from build123d import *

# Parameters (mm, degrees)
SKETCH_1_W                       = 120
SKETCH_1_H                       = 88
SKETCH_1_R                       = 32.5
SM_BASE_FLANGE_1_DEPTH           = 6
SM_EDGE_FLANGE_5_STRIP_W         = 36
SM_EDGE_FLANGE_5_STRIP_H         = 6
SM_EDGE_FLANGE_5_STRIP_CUT_DEPTH = 88
SM_EDGE_FLANGE_5_DEPTH           = 88
SM_EDGE_FLANGE_7_DEPTH           = 108
OTHER_START                      = -12
OTHER_1_OUTLINE_W                = 12
OTHER_1_OUTLINE_H                = 63
OTHER_1_DEPTH                    = 6
OTHER_START_2                    = -5
OTHER_1_2_OUTLINE_W              = 6
OTHER_1_2_OUTLINE_H              = 63
OTHER_1_2_DEPTH                  = 5
CHAMFER_1_SIZE                   = 25
MOVE_START                       = -12
MOVE_BODY_1_DEPTH                = 100
MOVE_START_2                     = -5
MOVE_BODY_1_2_OUTLINE_W          = 108
MOVE_BODY_1_2_OUTLINE_H          = 12
MOVE_BODY_1_2_OUTLINE_W_2        = 6
MOVE_BODY_1_2_OUTLINE_H_2        = 63
MOVE_BODY_1_2_DEPTH              = 93
MOVE_BODY_1_3_DEPTH              = 6
MOVE_BODY_1_4_DEPTH              = 88
MOVE_START_3                     = -6
MOVE_BODY_1_5_OUTLINE_W          = 108
MOVE_BODY_1_5_OUTLINE_H          = 12
MOVE_BODY_1_5_DEPTH              = 1
MOVE_BODY_1_6_OUTLINE_R          = 32.5
MOVE_BODY_1_6_DEPTH              = 12
MOVE_BODY_1_7_DEPTH              = 108


with BuildPart() as part:
    # Базовая кромка1: sheet metal written as solids
    # Sketch 1 → Базовая кромка1 (new body)
    with BuildSketch(Plane.XY):
        with Locations((60, 44)):
            Rectangle(SKETCH_1_W, SKETCH_1_H)
        with Locations((60, 38)):
            Circle(SKETCH_1_R, mode=Mode.SUBTRACT)
    extrude(amount=-SM_BASE_FLANGE_1_DEPTH)

    # Ребро-кромка5: sheet metal written as solids
    # Ребро-кромка5 strip (on a plane across the edge) → Ребро-кромка5 strip cut (cut)
    with BuildSketch(Plane(origin=(120, 0, 0), x_dir=(-1, 0, 0), z_dir=(0, 1, 0))):
        with Locations((-6, -3)):
            Rectangle(SM_EDGE_FLANGE_5_STRIP_W, SM_EDGE_FLANGE_5_STRIP_H)
    extrude(amount=SM_EDGE_FLANGE_5_STRIP_CUT_DEPTH, mode=Mode.SUBTRACT)

    # Ребро-кромка5 section (on a plane across the edge) → Ребро-кромка5 (add)
    with BuildSketch(Plane(origin=(120, 0, 0), x_dir=(-1, 0, 0), z_dir=(0, 1, 0))):
        with BuildLine():
            Line((0, 6), (0, 69))
            Line((0, 69), (6, 69))
            Line((6, 69), (6, 6))
            ThreePointArc((6, 6), (7.757359313, 1.757359313), (12, 0))
            Line((12, 0), (12, -6))
            ThreePointArc((12, -6), (3.514718626, -2.485281374), (0, 6))
        make_face()
    extrude(amount=SM_EDGE_FLANGE_5_DEPTH)

    # Ребро-кромка7: sheet metal written as solids
    # Ребро-кромка7 section (on a plane across the edge) → Ребро-кромка7 (add)
    with BuildSketch(Plane(origin=(0, -6, 0), x_dir=(0, 1, 0), z_dir=(1, 0, 0))):
        with BuildLine():
            Line((-6, 6), (-6, 69))
            Line((-6, 69), (0, 69))
            Line((0, 69), (0, 6))
            ThreePointArc((0, 6), (1.757359313, 1.757359313), (6, 0))
            Line((6, 0), (6, -6))
            ThreePointArc((6, -6), (-2.485281374, -2.485281374), (-6, 6))
        make_face()
    extrude(amount=SM_EDGE_FLANGE_7_DEPTH)

    # Other 1: read off the stored shape, not the designer's step
    # Other 1 outline → Other 1 (add)
    with BuildSketch(Plane(origin=(0, 0, 0), x_dir=(1, 0, 0), z_dir=(0, 1, 0)).offset(OTHER_START)):
        with Locations((114, -37.5)):
            Rectangle(OTHER_1_OUTLINE_W, OTHER_1_OUTLINE_H)
    extrude(amount=OTHER_1_DEPTH)

    # Other 1 2 outline → Other 1 2 (add)
    with BuildSketch(Plane(origin=(0, 0, 0), x_dir=(1, 0, 0), z_dir=(0, 1, 0)).offset(OTHER_START_2)):
        with Locations((117, -37.5)):
            Rectangle(OTHER_1_2_OUTLINE_W, OTHER_1_2_OUTLINE_H)
    extrude(amount=OTHER_1_2_DEPTH)

    # Фаска1
    chamfer_1_edges = [part.edges().sort_by_distance(p)[0] for p in [
        (0, -9, 69),
        (0, 88, -3),
    ]]
    chamfer(chamfer_1_edges, length=CHAMFER_1_SIZE)

    # Move Body 1: read off the stored shape, not the designer's step
    # Move Body 1 outline → Move Body 1 (cut)
    with BuildSketch(Plane(origin=(0, 0, 0), x_dir=(1, 0, 0), z_dir=(0, 1, 0)).offset(MOVE_START)):
        with BuildLine():
            Line((0, -6), (0, -44))
            Line((0, -44), (25, -69))
            Line((25, -69), (120, -69))
            Line((120, -69), (120, -6))
            ThreePointArc((120, -6), (119.591109915, -2.894171459), (118.392304845, 0))
            ThreePointArc((118.392304845, 0), (116.40755123, -2.562305899), (113.809475019, -4.5))
            ThreePointArc((113.809475019, -4.5), (113.952178178, -5.243974245), (114, -6))
            Line((114, -6), (0, -6))
        make_face()
        with BuildLine():
            Line((108, 6), (108, 0))
            ThreePointArc((108, 0), (111.674234614, 1.25658351), (113.809475019, 4.5))
            ThreePointArc((113.809475019, 4.5), (111, 5.618950038), (108, 6))
        make_face()
    extrude(amount=MOVE_BODY_1_DEPTH, mode=Mode.SUBTRACT)

    # Move Body 1 2 outline → Move Body 1 2 (add)
    with BuildSketch(Plane(origin=(0, 0, 0), x_dir=(1, 0, 0), z_dir=(0, 1, 0)).offset(MOVE_START_2)):
        with Locations((54, 0)):
            Rectangle(MOVE_BODY_1_2_OUTLINE_W, MOVE_BODY_1_2_OUTLINE_H)
        with Locations((117, 37.5)):
            Rectangle(MOVE_BODY_1_2_OUTLINE_W_2, MOVE_BODY_1_2_OUTLINE_H_2)
    extrude(amount=MOVE_BODY_1_2_DEPTH)

    # Move Body 1 3 outline → Move Body 1 3 (add)
    with BuildSketch(Plane(origin=(0, 0, 0), x_dir=(1, 0, 0), z_dir=(0, 1, 0)).offset(MOVE_START)):
        Polygon((0, -6), (108, -6), (108, 6), (120, 6), (120, 69), (25, 69), (0, 44), align=None)
    extrude(amount=MOVE_BODY_1_3_DEPTH)

    # Move Body 1 4 outline → Move Body 1 4 (add)
    with BuildSketch(Plane(origin=(0, 0, 0), x_dir=(1, 0, 0), z_dir=(0, 1, 0))):
        with BuildLine():
            Line((108, 0), (108, -6))
            ThreePointArc((108, -6), (111, -5.618950038), (113.809475019, -4.5))
            ThreePointArc((113.809475019, -4.5), (111.674234614, -1.25658351), (108, 0))
        make_face()
        with BuildLine():
            ThreePointArc((113.809475019, 4.5), (116.40755123, 2.562305899), (118.392304845, 0))
            ThreePointArc((118.392304845, 0), (119.591109915, 2.894171459), (120, 6))
            Line((120, 6), (114, 6))
            ThreePointArc((114, 6), (113.952178178, 5.243974245), (113.809475019, 4.5))
        make_face()
    extrude(amount=MOVE_BODY_1_4_DEPTH)

    # Move Body 1 5 outline → Move Body 1 5 (add)
    with BuildSketch(Plane(origin=(0, 0, 0), x_dir=(1, 0, 0), z_dir=(0, 1, 0)).offset(MOVE_START_3)):
        with Locations((54, 0)):
            Rectangle(MOVE_BODY_1_5_OUTLINE_W, MOVE_BODY_1_5_OUTLINE_H)
    extrude(amount=MOVE_BODY_1_5_DEPTH)

    # Move Body 1 6 outline → Move Body 1 6 (cut)
    with BuildSketch(Plane.XY.offset(MOVE_START_3)):
        with Locations((60, 38)):
            Circle(MOVE_BODY_1_6_OUTLINE_R)
        Polygon((0, 88), (0, 63), (25, 88), align=None)
    extrude(amount=MOVE_BODY_1_6_DEPTH, mode=Mode.SUBTRACT)

    # Move Body 1 7 outline → Move Body 1 7 (cut)
    with BuildSketch(Plane.YZ):
        with BuildLine():
            Line((88, -6), (88, 0))
            Line((88, 0), (0, 0))
            ThreePointArc((0, 0), (-4.242640687, -1.757359313), (-6, -6))
            Line((-6, -6), (88, -6))
        make_face()
        with BuildLine():
            ThreePointArc((-12, -6), (-8.485281374, 2.485281374), (0, 6))
            Line((0, 6), (-12, 6))
            Line((-12, 6), (-12, -6))
        make_face()
    extrude(amount=MOVE_BODY_1_7_DEPTH, mode=Mode.SUBTRACT)


solid = part.part
Geometry: final body of the model. Coordinates: model frame, mm. A direction names the side the tool comes from. Give positions to 0.01 mm unless a question says otherwise; leave off trailing zeros. Loops run counter-clockwise (first coordinate to the right, second up) from the corner with the lowest first, then second, coordinate; pieces in that order, holes last. Notation, with made-up numbers: M 18.5,62.5 L 47.5,62.5 A32 cw 47.5,89.5 Z; hole C -34.75,79 d4. An arc over 180 degrees is marked long. Put each result on its own line as item: value.
1) Cut plane A-A, the plane x = 60. Return the cut outline in (y, z).
Computed values:
outline: M -12,-69 L -6,-69 L -6,-6 A6 cw 0,0 L 5.5,0 L 5.5,6 L 0,6 A12 ccw -12,-6 Z; M 70.5,0 L 88,0 L 88,6 L 70.5,6 Z
2) First-contact query: P1, Ø4, axis at x = 118.5, y = -1.5, coming from the +Z side; P2, Ø6.5, axis at x = 115, y = -7.5, coming from the +Z side; P3, Ø9.5, axis at x = 111, z = 0.5, coming from the -Y side. Flat tips, straight axial feed; report the tip coordinate or a pass-through.
Computed values:
P1: stops at z = 1.73
P2: stops at z = -6
P3: stops at y = -11.66
3) Reachability of faces 1 (the flat face through (29, 54, 0)), 2 (the flat face through (59, -12, -38)), 3 (the flat face through (108, -6, 0)) from +Z, -Z, +X, -X, +Y, -Y: full face, straight path, thin tool, end or side. Return the list, or none.
Computed values:
face 1: -Z, -X, +Y
face 2: +Z, -Z, +X, -X, -Y
face 3: +Z, +X, -Y
4) Cut plane D-D, the plane y = 3. Return the cut outline in (x, z), plus the area to 3 significant figures.
Computed values:
outline: M 0,0 L 108,0 A6 cw 114,-6 L 114,-69 L 120,-69 L 120,-6 A12 ccw 108,6 L 0,6 Z
area: 1,110 mm^2
5) Mould query, pull axis Y, two halves, no side actions, for faces 4 (the flat face through (29, 53, 6)), 5 (the flat face through (93, 88, 2)), 6 (the flat face through (117, -5, -38)), 7 (the cylindrical face through (27.53, 39.43, 2.96)). Classes: released by +Y, released by -Y, zero draft, split by the parting line, or undercut.
Computed values:
face 4: zero draft
face 5: released by +Y
face 6: undercut
face 7: undercut
6) Cut plane C-C, the plane z = -61. Return the cut outline in (x, y), plus the area to 3 significant figures.
Computed values:
outline: M 17,-12 L 120,-12 L 120,-6 L 17,-6 Z; M 114,-5 L 120,-5 L 120,88 L 114,88 Z
area: 1,180 mm^2
7) Material intervals for L1, parallel to Z at x = 83, y = 1; L2, parallel to Y at x = 61.5, z = -33.5; L3, parallel to X at y = 38, z = 2.4, sorted ascending. Write a range as from..to.
Computed values:
L1: z = 0..6
L2: y = -12..-6
L3: x = 0..27.5, 92.5..116.57
8) Cut plane B-B, the plane y = 38. Return the cut outline in (x, z).
Computed values:
outline: M 0,0 L 27.5,0 L 27.5,6 L 0,6 Z; M 92.5,0 L 108,0 A6 cw 114,-6 L 114,-69 L 120,-69 L 120,-6 A12 ccw 108,6 L 92.5,6 Z
